from build123d import *

# Parameters (mm, degrees)
F0_R     = 3.75
F1_DEPTH = 9.375
F2_W     = 25
F2_H     = 9.525
F3_DEPTH = 25
F4_R     = 2.283414
F5_DEPTH = 9.525


with BuildPart() as f1:
    # F0 (on Top) → F1 (new body)
    with BuildSketch(Plane.XY):
        with BuildLine():
            Line((0, 150), (0, 0))
            Line((0, 0), (25, 0))
            Line((25, 0), (25, 150))
            ThreePointArc((25, 150), (12.5, 162.5), (0, 150))
        make_face()
        with Locations((12.5, 150)):
            Circle(F0_R, mode=Mode.SUBTRACT)
    extrude(amount=F1_DEPTH)

    # F2 (on face) → F3 (join)
    with BuildSketch(Plane.XY.offset(9.375)):
        with Locations((12.5, 4.7625)):
            Rectangle(F2_W, F2_H)
    extrude(amount=F3_DEPTH)

    # F4 (on face) → F5 (cut, through all)
    with BuildSketch(Plane(origin=(0, 9.525, 0), x_dir=(-1, 0, 0), z_dir=(0, 1, 0))):
        with Locations((-12.5, 20)):
            Circle(F4_R)
    extrude(amount=-F5_DEPTH, mode=Mode.SUBTRACT)


solid = f1.part
Geometry check sheet. Reference: the model listing, model coordinates, mm. Give positions to 0.01 mm unless a question says otherwise; leave off trailing zeros. Loops run counter-clockwise (first coordinate to the right, second up) from the corner with the lowest first, then second, coordinate; pieces in that order, holes last.
(1) Release check for a two-part mould opening along Y. For faces 1 (the cylindrical face through (11.69, 146.34, 4.62)), 2 (the flat face through (12, 9.525, 24)), 3 (the flat face through (12, 87, 9.375)) record: released by +Y, released by -Y, zero draft, split by the parting line, or undercut.
From the geometry:
face 1: undercut
face 2: released by +Y
face 3: zero draft
(2) Section check C-C on y = 112. Record the cut outline in (x, z) (3 decimals), then the cut area to 3 significant figures.
From the geometry:
outline: (0, 0) - (25, 0) - (25, 9.375) - (0, 9.375) - close
area: 234 mm2
(3) Section check D-D on z = 27.5. Record the cut outline in (x, y) (3 decimals), then the cut area to 3 significant figures.
From the geometry:
outline: (0, 0) - (25, 0) - (25, 9.525) - (0, 9.525) - close
area: 238 mm2
(4) Section check B-B on x = 12.5. Record the cut outline in (y, z) (3 decimals), then the cut area to 3 significant figures.
From the geometry:
outline: (0, 0) - (146.25, 0) - (146.25, 9.375) - (9.525, 9.375) - (9.525, 17.717) - (0, 17.717) - close; (0, 22.283) - (9.525, 22.283) - (9.525, 34.375) - (0, 34.375) - close; (153.75, 0) - (162.5, 0) - (162.5, 9.375) - (153.75, 9.375) - close
area: 1,650 mm2
(5) Section check A-A on z = 20. Record the cut outline in (x, y) (3 decimals), then the cut area to 3 significant figures.
From the geometry:
outline: (0, 0) - (10.217, 0) - (10.217, 9.525) - (0, 9.525) - close; (14.783, 0) - (25, 0) - (25, 9.525) - (14.783, 9.525) - close
area: 195 mm2
(6) Thickness scan on L1, parallel to Y at x = 12.5, z = 6; L2, parallel to Y at x = 8.5, z = 29.5 (3 decimals); L3, parallel to X at y = 150, z = 3. Record the ranges inside material, lowest first.
From the geometry:
L1: y = 0 to 146.25, 153.75 to 162.5
L2: y = 0 to 9.525
L3: x = 0 to 8.75, 16.25 to 25
(7) Depth check by flat-ended pin: pin 1 Ø8 at (x, y) = (10.5, 120) entering from +Z (3 decimals); pin 2 Ø1.5 at (x, z) = (21.5, 9.5) entering from +Y. Enter the tip coordinate at first touch or a pass-through.
From the geometry:
pin 1: stops at z = 9.375
pin 2: stops at y = 159.38
